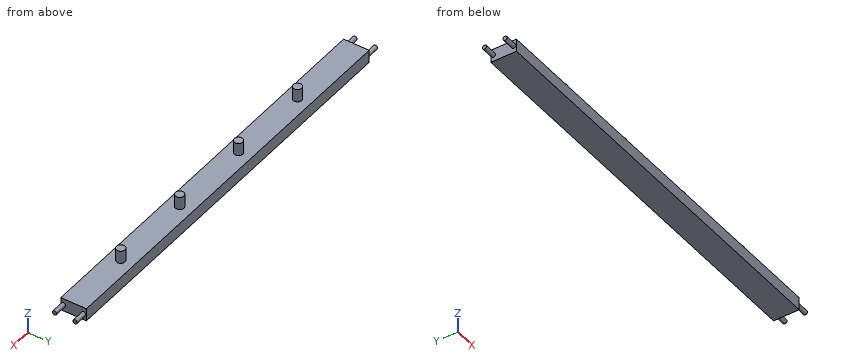
from build123d import *

# Parameters (mm, degrees)
F0_W     = 1219.2
F0_H     = 76.2
F1_DEPTH = 38.1
F2_R     = 12.7
F3_DEPTH = 38.1
F5_DEPTH = 38.1
F7_DEPTH = 38.1


with BuildPart() as f1:
    # F0 (on Top) → F1 (new body)
    with BuildSketch(Plane.XY):
        with Locations((464.734342, -10.029948)):
            Rectangle(F0_W, F0_H)
    extrude(amount=F1_DEPTH)

    # F2 (on face) → F3 (join)
    with BuildSketch(Plane.XY.offset(38.1)):
        with Locations((109.134342, -10.029948)):
            Circle(F2_R)
        with Locations((363.134342, -10.029948)):
            Circle(F2_R)
        with Locations((617.134342, -10.029948)):
            Circle(F2_R)
        with Locations((871.134342, -10.029948)):
            Circle(F2_R)
    extrude(amount=F3_DEPTH)

    # F4 (on face) → F5 (join)
    with BuildSketch(Plane(origin=(-144.865658, 0, 0), x_dir=(0, -1, 0), z_dir=(-1, 0, 0))):
        with BuildLine():
            ThreePointArc((-14.100052, 19.05), (-20.450052, 25.4), (-26.800052, 19.05))
            Line((-26.800052, 19.05), (-14.100052, 19.05))
        make_face()
        with BuildLine():
            ThreePointArc((46.859948, 19.05), (40.509948, 25.4), (34.159948, 19.05))
            Line((34.159948, 19.05), (46.859948, 19.05))
        make_face()
        with BuildLine():
            Line((46.859948, 19.05), (34.159948, 19.05))
            ThreePointArc((34.159948, 19.05), (40.509948, 12.7), (46.859948, 19.05))
        make_face()
        with BuildLine():
            Line((-14.100052, 19.05), (-26.800052, 19.05))
            ThreePointArc((-26.800052, 19.05), (-20.450052, 12.7), (-14.100052, 19.05))
        make_face()
    extrude(amount=F5_DEPTH)

    # F6 (on face) → F7 (join)
    with BuildSketch(Plane.YZ.offset(1074.334342)):
        with BuildLine():
            ThreePointArc((-34.159948, 19.05), (-40.509948, 25.4), (-46.859948, 19.05))
            Line((-46.859948, 19.05), (-34.159948, 19.05))
        make_face()
        with BuildLine():
            ThreePointArc((26.800052, 19.05), (20.450052, 25.4), (14.100052, 19.05))
            Line((14.100052, 19.05), (26.800052, 19.05))
        make_face()
        with BuildLine():
            Line((26.800052, 19.05), (14.100052, 19.05))
            ThreePointArc((14.100052, 19.05), (20.450052, 12.7), (26.800052, 19.05))
        make_face()
        with BuildLine():
            Line((-34.159948, 19.05), (-46.859948, 19.05))
            ThreePointArc((-46.859948, 19.05), (-40.509948, 12.7), (-34.159948, 19.05))
        make_face()
    extrude(amount=F7_DEPTH)


solid = f1.part
Part model, mm, in its own coordinate system. Coordinates: 2 decimals unless noted, no trailing zeros. Loops run counter-clockwise (first coordinate to the right, second up) from the corner with the lowest first, then second, coordinate; pieces in that order, holes last. Notation, with made-up numbers: (6, 77) -> (22, 77) arc R25 cw to (22, 104) -> close; hole circle Ø7 at (73, 63). An arc over 180 degrees is marked (long way). Use a Markdown table: item, result. Add a question column.
Item 1: Probe probe 1 along X at (y, z) = (-12.5, 64.5); probe 2 along Z at (x, y) = (-57, -35.5); probe 3 along X at (y, z) = (-14, 65). List the from-to ranges inside material, lowest first.
Item 2: Band-saw the part on A-A on x = 465.5. Write the cut outline in (y, z).
Item 3: Flat gauge pins, fed straight in: P1, Ø4, axis at y = -3.5, z = 10.5, coming from the +X side; P2, Ø2, axis at x = 629.5, y = -24, coming from the +Z side; P3, Ø3, axis at y = -9, z = 40, coming from the -X side. Where does each tip first touch, or does it go through?
Item 4: Band-saw the part on B-B on z = 53. Write the cut outline in (x, y), plus the area to 3 significant figures.
Geometry says:
| question | item | result |
|---|---|---|
| 1 | probe 1 | 96.68 to 121.59, 350.68 to 375.59, 604.68 to 629.59, 858.68 to 883.59 |
| 1 | probe 2 | 0 to 38.1 |
| 1 | probe 3 | 97.07 to 121.2, 351.07 to 375.2, 605.07 to 629.2, 859.07 to 883.2 |
| 2 | outline | (-48.13, 0) -> (28.07, 0) -> (28.07, 38.1) -> (-48.13, 38.1) -> close |
| 3 | P1 | x = 1074.33 |
| 3 | P2 | z = 38.1 |
| 3 | P3 | x = 96.43 |
| 4 | outline | circle Ø25.4 at (109.13, -10.03); circle Ø25.4 at (363.13, -10.03); circle Ø25.4 at (617.13, -10.03); circle Ø25.4 at (871.13, -10.03) |
| 4 | area | 2,030 mm² |
